Geometry: see drawing. Coordinates: mm, zero at the bounding-box minimum. Give positions to 0.01 mm unless a question says otherwise; leave off trailing zeros. Order: outer loops, then holes, each group sorted by start corner. A loop starts at its lowest first (then second) coordinate and runs counter-clockwise, first axis right, second up. Notation, with made-up numbers: (1.25, 33.25) - (56.25, 33.25) arc R22 cw to (56.25, 64.25) - close; hole circle Ø7 at (49.25, 76.25). An arc over 180 degrees is marked (long way). Put each result on its own line as item: value. Start each with the question number.
1. Section A-A on x = 187.5. Return the cut outline in (y, z).
2. Ray query, line 1 along Z through (x, y) = (162.5, 2.95); line 2 along Z through (x, y) = (110, 0.95). Return the intervals inside material, ascending. Write a range as from..to.
3. Section B-B on z = 87.5. Count the separate pieces of the cut face and the enclosed holes in it, plus the area to 3 significant figures.
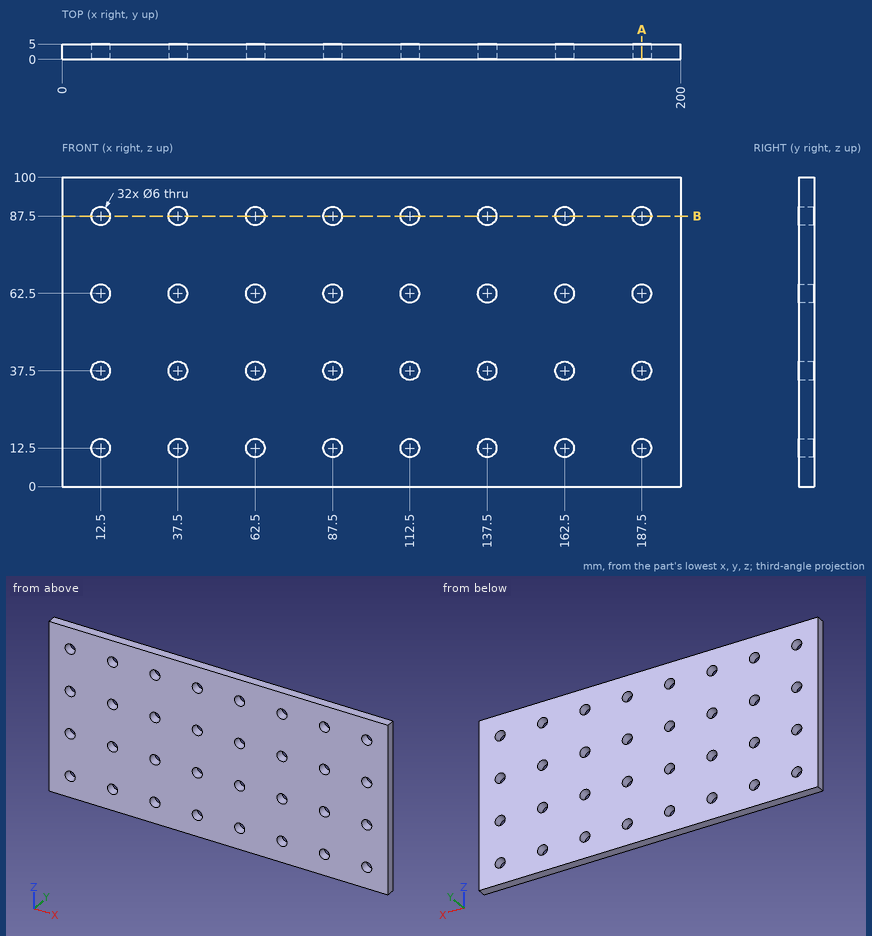
Resolved:
1. outline: (0, 0) - (5, 0) - (5, 9.5) - (0, 9.5) - close; (0, 15.5) - (5, 15.5) - (5, 34.5) - (0, 34.5) - close; (0, 40.5) - (5, 40.5) - (5, 59.5) - (0, 59.5) - close; (0, 65.5) - (5, 65.5) - (5, 84.5) - (0, 84.5) - close; (0, 90.5) - (5, 90.5) - (5, 100) - (0, 100) - close
2. line 1: 0..9.5, 15.5..34.5, 40.5..59.5, 65.5..84.5, 90.5..100
2. line 2: 0..10.84, 14.16..35.84, 39.16..60.84, 64.16..85.84, 89.16..100
3. separate pieces: 9
3. enclosed holes: 0
3. area: 760 mm^2
